```python
from build123d import *

# Parameters (mm, degrees)
SKETCH1_R           = 63.5
BASE_DEPTH          = 12.7
MOUNT_DEPTH         = 25.4
FILLET1_RADIUS      = 25.4
FILLET1_LENGTH      = 12.7
FILLET2_RADIUS      = 25.4
FILLET2_LENGTH      = 12.7
PIN_HOLE_DEPTH      = 118.774954893
PIN_HOLE_DEPTH_BACK = 118.774954893
SKETCH3_R           = 9.525
SKETCH4_R           = 6.35
BOLT_PATTERN_DEPTH  = 110.985226281
FILLET3_R           = 3.81
CHAMFER1_SIZE       = 3.81


with BuildPart() as part:
    # Sketch1 → Base (new body)
    with BuildSketch(Plane(origin=(0, 0, 0), x_dir=(1, 0, 0), z_dir=(0, 1, 0))):
        with Locations(Location((0, 0, 0), (0, 0, 270))):
            Circle(SKETCH1_R)
    extrude(amount=BASE_DEPTH)

    # Sketch2 → Mount (add, symmetric)
    with BuildSketch(Plane.XY):
        Polygon((-12.7, 25.4), (12.7, 25.4), (12.7, 76.2), (25.4, 76.2), (25.4, 12.7), (-25.4, 12.7), (-25.4, 76.2), (-12.7, 76.2), align=None)
    extrude(amount=MOUNT_DEPTH, both=True)

    # Fillet1: full round fillet: the end face becomes a half cylinder, R = half its width
    fillet1_face = Plane((19.05, 76.2, 0), x_dir=(-1, 0, 0), z_dir=(0, 1, 0))  # on the end face: x along it, z out of the body
    fillet1_slab = fillet1_face.offset(-FILLET1_RADIUS / 2) * Box(FILLET1_LENGTH, 2 * FILLET1_RADIUS, FILLET1_RADIUS, mode=Mode.PRIVATE)  # the body's end, R deep
    fillet1_round = Plane((19.05, 50.8, 0), x_dir=(0, 1, 0), z_dir=(-1, 0, 0)) * Cylinder(FILLET1_RADIUS, FILLET1_LENGTH, mode=Mode.PRIVATE)  # its axis R under the face
    add(fillet1_slab - fillet1_round, mode=Mode.SUBTRACT)

    # Fillet2: full round fillet: the end face becomes a half cylinder, R = half its width
    fillet2_face = Plane((-19.05, 76.2, 0), x_dir=(1, 0, 0), z_dir=(0, 1, 0))  # on the end face: x along it, z out of the body
    fillet2_slab = fillet2_face.offset(-FILLET2_RADIUS / 2) * Box(FILLET2_LENGTH, 2 * FILLET2_RADIUS, FILLET2_RADIUS, mode=Mode.PRIVATE)  # the body's end, R deep
    fillet2_round = Plane((-19.05, 50.8, 0), x_dir=(0, 1, 0), z_dir=(1, 0, 0)) * Cylinder(FILLET2_RADIUS, FILLET2_LENGTH, mode=Mode.PRIVATE)  # its axis R under the face
    add(fillet2_slab - fillet2_round, mode=Mode.SUBTRACT)

    # Sketch3 → Pin Hole (cut, two sides: drawn at the far end of the back side and taken through both)
    with BuildSketch(Plane(origin=(0, 0, 0), x_dir=(0, 0, -1), z_dir=(1, 0, 0)).offset(-PIN_HOLE_DEPTH_BACK)):
        with Locations((0, 50.8)):
            Circle(SKETCH3_R)
    extrude(amount=PIN_HOLE_DEPTH + PIN_HOLE_DEPTH_BACK, mode=Mode.SUBTRACT)

    # Sketch4 → Bolt Pattern (cut, through all)
    with BuildSketch(Plane(origin=(0, 12.7, 0), x_dir=(1, 0, 0), z_dir=(0, 1, 0))):
        with Locations(Location((0, -44.45, 0), (0, 0, 270))):
            Circle(SKETCH4_R)
        with Locations(Location((-44.45, 0, 0), (0, 0, 270))):
            Circle(SKETCH4_R)
        with Locations(Location((0, 44.45, 0), (0, 0, 270))):
            Circle(SKETCH4_R)
        with Locations(Location((44.45, 0, 0), (0, 0, 270))):
            Circle(SKETCH4_R)
    extrude(amount=-BOLT_PATTERN_DEPTH, mode=Mode.SUBTRACT)

    # Fillet3
    fillet3_edges = [part.edges().sort_by_distance(p)[0] for p in [
        (25.4, 12.7, 0),
        (0, 12.7, 25.4),
        (0, 12.7, -25.4),
        (-25.4, 12.7, 0),
    ]]
    fillet(fillet3_edges, radius=FILLET3_R)

    # Chamfer1
    chamfer1_edges = [part.edges().sort_by_distance(p)[0] for p in [
        (0, 12.7, -63.5),
    ]]
    chamfer(chamfer1_edges, length=CHAMFER1_SIZE)


solid = part.part
```
Verification items for the finished model (mm, model axes). A direction names the side the tool comes from. Round coordinates to 2 decimals unless told otherwise and drop trailing zeros. Write each loop counter-clockwise with the first axis right and the second up, starting at its lowest first coordinate (ties: lowest second). Pieces come first, ordered by that corner, then holes. Notation, with made-up numbers: (12.25, -20.5) -> (56.25, -20.5) arc R9 ccw to (56.25, -12.5) -> close; hole circle Ø2 at (-6, -32.75). An arc over 180 degrees is marked (long way). Write each question's results on one line, items separated by ' | '. Start each with the question number.
1. Cross-section at B-B (x = 0). Enter the section's corners in (y, z), then the cut area to 3 significant figures.
2. Depth check by flat-ended pin: P1, Ø25, axis at y = 50.8, z = 0, coming from the -X side; P2, Ø6, axis at x = 47.5, z = 27.5, coming from the +Y side; P3, Ø15, axis at y = 53, z = -11, coming from the +X side; P4, Ø10, axis at x = 0, z = 44.45, coming from the +Y side. Enter the tip coordinate at first touch or a pass-through.
3. Material ranges on probe 1 along X at (y, z) = (5.25, 0); probe 2 along X at (y, z) = (64, 8.5); probe 3 along Z at (x, y) = (21, 50.8) (3 decimals), recorded low to high. Write a range as from..to.
4. Draft check along Z on faces 4 (the flat face through (-39, 12.7, 12)), 5 (the cylindrical face through (1.907, 6.439, -38.393)), 6 (the flat face through (0, 22, -25.4)). Enter one of: +Z half, -Z half, draft (parallel to the pull), parting line (faces both ways), or undercut.
5. Set-up check for faces 1 (the flat face through (25.4, 40, 0)), 2 (the flat face through (0, 22, 25.4)), 3 (the flat face through (-25.4, 39, 0)): record each of +Z, -Z, +X, -X, +Y, -Y from which the full face is reachable in a straight line by a thin tool's end or side.
6. Cross-section at A-A (z = 0). Count the separate pieces of the cut face and the enclosed holes in it, then the cut area to 3 significant figures.
7. Cross-section at D-D (y = 67). Enter the section's corners in (x, z), then the cut area to 3 significant figures.
8. Cross-section at C-C (y = 37). Enter the section's corners in (x, z).
Solutions:
1) outline: (0, -63.5) -> (8.89, -63.5) -> (12.7, -59.69) -> (12.7, -50.8) -> (0, -50.8) -> close; (0, -38.1) -> (12.7, -38.1) -> (12.7, -29.21) arc R3.81 cw to (16.51, -25.4) -> (25.4, -25.4) -> (25.4, 25.4) -> (16.51, 25.4) arc R3.81 cw to (12.7, 29.21) -> (12.7, 38.1) -> (0, 38.1) -> close; (0, 50.8) -> (12.7, 50.8) -> (12.7, 59.69) -> (8.89, 63.5) -> (0, 63.5) -> close | area: 1,930 mm2
2) P1: stops at x = -25.4 | P2: stops at y = 12.7 | P3: stops at x = 25.4 | P4: passes through
3) probe 1: x = -63.5..-50.8, -38.1..38.1, 50.8..63.5 | probe 2: x = -25.4..-12.7, 12.7..25.4 | probe 3: z = -25.4..-9.525, 9.525..25.4
4) face 4: draft | face 5: undercut | face 6: -Z half
5) face 1: +Z, -Z, +X, +Y | face 2: +Z, +X, -X, +Y | face 3: +Z, -Z, -X, +Y
6) separate pieces: 5 | enclosed holes: 0 | area: 2,730 mm2
7) outline: (-25.4, -19.56) -> (-12.7, -19.56) -> (-12.7, 19.56) -> (-25.4, 19.56) -> close; (12.7, -19.56) -> (25.4, -19.56) -> (25.4, 19.56) -> (12.7, 19.56) -> close | area: 994 mm2
8) outline: (-25.4, -25.4) -> (-12.7, -25.4) -> (-12.7, 25.4) -> (-25.4, 25.4) -> close; (12.7, -25.4) -> (25.4, -25.4) -> (25.4, 25.4) -> (12.7, 25.4) -> close
